Source: CAD feature listing. Evaluate the final solid. Frame: model axes, mm. A direction names the side the tool comes from. Coordinates: 2 decimals unless noted, no trailing zeros. Write each loop counter-clockwise with the first axis right and the second up, starting at its lowest first coordinate (ties: lowest second). Pieces come first, ordered by that corner, then holes. Notation, with made-up numbers: (27.5, 39.25) -> (76.5, 39.25) arc R19 cw to (76.5, 60.25) -> close; hole circle Ø9 at (82, 21.5). An arc over 180 degrees is marked (long way). Write item = value, one per line.
from build123d import *

# Parameters (mm, degrees)
SKETCH1_W           = 35.2
SKETCH1_H           = 35.2
BOSS_EXTRUDE1_DEPTH = 20
SKETCH2_R           = 11
BOSS_EXTRUDE2_DEPTH = 2
SKETCH3_R           = 2.5
BOSS_EXTRUDE3_DEPTH = 10.5
SKETCH4_R           = 1.5
CUT_EXTRUDE1_DEPTH  = 4.5
CHAMFER1_SIZE       = 3


with BuildPart() as part:
    # Sketch1 → Boss-Extrude1 (new body)
    with BuildSketch(Plane.XY):
        Rectangle(SKETCH1_W, SKETCH1_H)
    extrude(amount=BOSS_EXTRUDE1_DEPTH)

    # Sketch2 → Boss-Extrude2 (add)
    with BuildSketch(Plane.XY.offset(20)):
        Circle(SKETCH2_R)
    extrude(amount=BOSS_EXTRUDE2_DEPTH)

    # Sketch3 → Boss-Extrude3 (add)
    with BuildSketch(Plane.XY.offset(22)):
        with Locations(Location((0, 0, 0), (0, 0, 180))):
            Circle(SKETCH3_R)
    extrude(amount=BOSS_EXTRUDE3_DEPTH)

    # Sketch4 → Cut-Extrude1 (cut)
    with BuildSketch(Plane.XY.offset(20)):
        with Locations((13, 13)):
            Circle(SKETCH4_R)
        with Locations((13, -13)):
            Circle(SKETCH4_R)
        with Locations((-13, -13)):
            Circle(SKETCH4_R)
        with Locations((-13, 13)):
            Circle(SKETCH4_R)
    extrude(amount=-CUT_EXTRUDE1_DEPTH, mode=Mode.SUBTRACT)

    # Chamfer1
    chamfer1_edges = [part.edges().sort_by_distance(p)[0] for p in [
        (17.6, -17.6, 10),
        (-17.6, -17.6, 10),
        (-17.6, 17.6, 10),
        (17.6, 17.6, 10),
    ]]
    chamfer(chamfer1_edges, length=CHAMFER1_SIZE)


solid = part.part
1) Material intervals for probe 1 along Y at (x, z) = (-13, 18.2); probe 2 along Z at (x, y) = (-8, -13); probe 3 along Z at (x, y) = (-9.5, 2), sorted ascending. Write a range as [from, to].
Answer block:
probe_1 = [-17.6, -14.5], [-11.5, 11.5], [14.5, 17.6]
probe_2 = [0, 20]
probe_3 = [0, 22]
2) Cut plane D-D, the plane x = -6. Output: boundary loops of the cut face in (y, z).
Answer block:
outline = (-17.6, 0) -> (17.6, 0) -> (17.6, 20) -> (9.22, 20) -> (9.22, 22) -> (-9.22, 22) -> (-9.22, 20) -> (-17.6, 20) -> close
3) Cut plane A-A, the plane x = 0. Output: boundary loops of the cut face in (y, z).
Answer block:
outline = (-17.6, 0) -> (17.6, 0) -> (17.6, 20) -> (11, 20) -> (11, 22) -> (2.5, 22) -> (2.5, 32.5) -> (-2.5, 32.5) -> (-2.5, 22) -> (-11, 22) -> (-11, 20) -> (-17.6, 20) -> close
4) First-contact query: pin 1 Ø2.5 at (x, y) = (-13, -13) entering from +Z; pin 2 Ø3.5 at (x, y) = (12.5, -13) entering from +Z. Flat tips, straight axial feed; report the tip coordinate or a pass-through.
Answer block:
pin_1 = 15.5
pin_2 = 20
5) Pull-direction query (X, two-part tool) for faces 3 (the flat face through (16.1, 16.1, 9.9)), 4 (the flat face through (-13, -13, 15.5)), 5 (the flat face through (-3, 0, 22)), 6 (the flat face through (-16.1, -16.1, 9.9)); classes: +X half, -X half, draft (parallel to the pull), parting line (faces both ways), or undercut.
Answer block:
face_3 = +X half
face_4 = undercut
face_5 = draft
face_6 = -X half
6) Reachability of faces 1 (the flat face through (-8, -8, 20)), 2 (the flat face through (0, 0, 32.5)) from +Z, -Z, +X, -X, +Y, -Y: full face, straight path, thin tool, end or side. Return the list, or none.
Answer block:
face_1 = +Z
face_2 = +Z, +X, -X, +Y, -Y
7) Cut plane C-C, the plane z = 23. Output: boundary loops of the cut face in (x, y), and give its area (3 significant figures).
Answer block:
outline = circle Ø5 at (0, 0)
area = 19.6 mm2
